from build123d import *

# Parameters (mm, degrees)
F1_DEPTH = 12
F2_R     = 15
F3_DEPTH = 10
F4_R     = 14.5
F5_DEPTH = 11


with BuildPart() as f1:
    # F0 (on Front) → F1 (new body)
    with BuildSketch(Plane.XZ):
        with BuildLine():
            ThreePointArc((-87.5, -28.3037), (-84.571068, -35.374768), (-77.5, -38.3037))
            Line((-77.5, -38.3037), (22.5, -38.3037))
            ThreePointArc((22.5, -38.3037), (29.571068, -35.374768), (32.5, -28.3037))
            Line((32.5, -28.3037), (32.5, 31.6963))
            ThreePointArc((32.5, 31.6963), (29.571068, 38.767368), (22.5, 41.6963))
            Line((22.5, 41.6963), (-77.5, 41.6963))
            ThreePointArc((-77.5, 41.6963), (-84.571068, 38.767368), (-87.5, 31.6963))
            Line((-87.5, 31.6963), (-87.5, -28.3037))
        make_face()
    extrude(amount=F1_DEPTH)

    # F2 (on face) → F3 (cut)
    with BuildSketch(Plane.XZ.offset(12)):
        with BuildLine():
            Line((31, -28.3037), (31, 31.6963))
            ThreePointArc((31, 31.6963), (28.510408, 37.706708), (22.5, 40.1963))
            Line((22.5, 40.1963), (-77.5, 40.1963))
            ThreePointArc((-77.5, 40.1963), (-83.510408, 37.706708), (-86, 31.6963))
            Line((-86, 31.6963), (-86, -28.3037))
            ThreePointArc((-86, -28.3037), (-83.510408, -34.314108), (-77.5, -36.8037))
            Line((-77.5, -36.8037), (22.5, -36.8037))
            ThreePointArc((22.5, -36.8037), (28.510408, -34.314108), (31, -28.3037))
        make_face()
        with Locations((-61, 15.1963)):
            Circle(F2_R, mode=Mode.SUBTRACT)
        with Locations((6, 15.1963)):
            Circle(F2_R, mode=Mode.SUBTRACT)
    extrude(amount=-F3_DEPTH, mode=Mode.SUBTRACT)

    # F4 (on face) → F5 (cut)
    with BuildSketch(Plane(origin=(0, 0, 0), x_dir=(-1, 0, 0), z_dir=(0, 1, 0))):
        with Locations((-6, 15.1963)):
            Circle(F4_R)
    extrude(amount=-F5_DEPTH, mode=Mode.SUBTRACT)


solid = f1.part
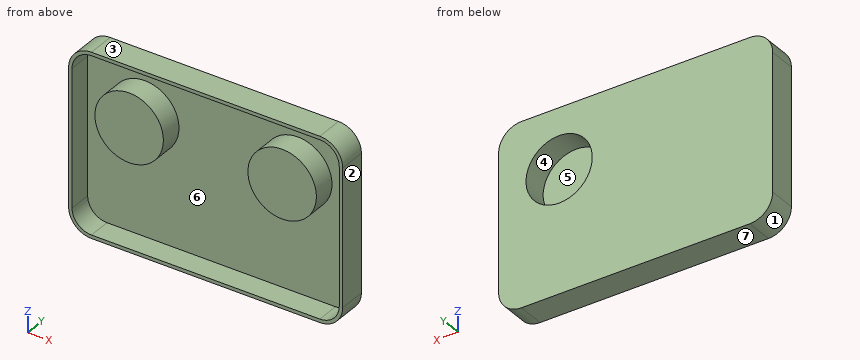
Could you check a few things on this model? Use its own coordinates, in mm. Face numbers are marked on the shaded views. A direction names the side the tool comes from. Round coordinates to 2 decimals unless told otherwise and drop trailing zeros. Write each loop counter-clockwise with the first axis right and the second up, starting at its lowest first coordinate (ties: lowest second). Pieces come first, ordered by that corner, then holes. Notation, with made-up numbers: (16.25, 33) - (63.25, 33) arc R26 cw to (63.25, 64) - close; hole circle Ø6 at (55.25, 53.5). An arc over 180 degrees is marked (long way). Use a Markdown table: item, result.
Q1. I want a section at D-D (z = -32). List the corners of the cut face in (x, y) for me.
Output values:
| item | result |
|---|---|
| outline | (-86.79, -12) - (-85.15, -12) - (-85.15, -2) - (30.15, -2) - (30.15, -12) - (31.79, -12) - (31.79, 0) - (-86.79, 0) - close |
Q2. Please list where these lines run through material, in increasing order: L1, parallel to Z at x = -60.5, y = -5; L2, parallel to Z at x = 6, y = -4; L3, parallel to X at y = -6.5, z = 15.
Output values:
| item | result |
|---|---|
| L1 | -38.3 to -36.8, 0.2 to 30.19, 40.2 to 41.7 |
| L2 | -38.3 to -36.8, 0.2 to 0.7, 29.7 to 30.2, 40.2 to 41.7 |
| L3 | -87.5 to -86, -76 to -46, -9 to -8.5, 20.5 to 21, 31 to 32.5 |
Q3. I want a section at A-A (x = 6). List the corners of the cut face in (y, z) for me, plus the area to 3 significant figures.
Output values:
| item | result |
|---|---|
| outline | (-12, -38.3) - (0, -38.3) - (0, 0.7) - (-11, 0.7) - (-11, 29.7) - (0, 29.7) - (0, 41.7) - (-12, 41.7) - (-12, 40.2) - (-2, 40.2) - (-2, 30.2) - (-12, 30.2) - (-12, 0.2) - (-2, 0.2) - (-2, -36.8) - (-12, -36.8) - close |
| area | 171 mm2 |
Q4. For pin 1 (2 mm diameter, centred on x = -54.5, z = -1.5, fed in from -Y), with a flat end and sliding along its axis, tell me the tip position at first contact or that it passes through.
Output values:
| item | result |
|---|---|
| pin 1 | y = -2 |
Q5. I want a section at C-C (x = -61). List the corners of the cut face in (y, z) for me, plus the area to 3 significant figures.
Output values:
| item | result |
|---|---|
| outline | (-12, -38.3) - (0, -38.3) - (0, 41.7) - (-12, 41.7) - (-12, 40.2) - (-2, 40.2) - (-2, 30.2) - (-12, 30.2) - (-12, 0.2) - (-2, 0.2) - (-2, -36.8) - (-12, -36.8) - close |
| area | 490 mm2 |
Q6. Thinking about a two-plate mould opening in X: for the marked faces 1, 2, 3 and 4, which applies, released by +X, released by -X, zero draft, split by the parting line, or undercut?
Output values:
| item | result |
|---|---|
| face 1 | released by -X |
| face 2 | released by +X |
| face 3 | zero draft |
| face 4 | undercut |
Q7. I want a section at B-B (z = -4). List the corners of the cut face in (x, y) for me.
Output values:
| item | result |
|---|---|
| outline | (-87.5, -12) - (-86, -12) - (-86, -2) - (31, -2) - (31, -12) - (32.5, -12) - (32.5, 0) - (-87.5, 0) - close |
Q8. For the marked faces 5, 6 and 7, which set-ups out of +Z, -Z, +X, -X, +Y, -Y let a thin tool reach every point of the face, with its end or its side?
Output values:
| item | result |
|---|---|
| face 5 | +Y |
| face 6 | -Y |
| face 7 | -Z, +X, -X, +Y, -Y |
